Check sheet for the modelled part. Datum: model origin and axes. Units: mm. A direction names the side the tool comes from. Round coordinates to 2 decimals unless told otherwise and drop trailing zeros. Order: outer loops, then holes, each group sorted by start corner. A loop starts at its lowest first (then second) coordinate and runs counter-clockwise, first axis right, second up.
```python
from build123d import *

# Parameters (mm, degrees)
BOSS_EXTRUDE1_DEPTH = 3
SKETCH3_W           = 5
SKETCH3_H           = 3
CUT_EXTRUDE2_DEPTH  = 55.166410256
SKETCH4_W           = 3
SKETCH4_H           = 15
CUT_EXTRUDE3_DEPTH  = 55.166410256
SKETCH5_R           = 1.5
CUT_EXTRUDE4_DEPTH  = 55.166410256
SKETCH6_R           = 1.6
CUT_EXTRUDE5_DEPTH  = 55.166410256


with BuildPart() as part:
    # Sketch1 → Boss-Extrude1 (new body)
    with BuildSketch(Plane(origin=(0, 0, 0), x_dir=(1, 0, 0), z_dir=(0, 1, 0))):
        Polygon((-45, 27), (-22.5, 27), (-22.5, 30), (-7.5, 30), (-7.5, 27), (7.5, 27), (7.5, 30), (22.5, 30), (22.5, 27), (45, 27), (45, -27), (22.5, -27), (22.5, -30), (7.5, -30), (7.5, -27), (-7.5, -27), (-7.5, -30), (-22.5, -30), (-22.5, -27), (-45, -27), align=None)
    extrude(amount=BOSS_EXTRUDE1_DEPTH)

    # Sketch3 → Cut-Extrude2 (cut, through all)
    with BuildSketch(Plane(origin=(0, 3, 0), x_dir=(1, 0, 0), z_dir=(0, 1, 0))):
        with Locations((-34.25, -19.5)):
            Rectangle(SKETCH3_W, SKETCH3_H)
        with Locations((-36.79, 19.5)):
            Rectangle(SKETCH3_W, SKETCH3_H)
    extrude(amount=-CUT_EXTRUDE2_DEPTH, mode=Mode.SUBTRACT)

    # Sketch4 → Cut-Extrude3 (cut, through all)
    with BuildSketch(Plane(origin=(0, 3, 0), x_dir=(1, 0, 0), z_dir=(0, 1, 0))):
        Rectangle(SKETCH4_W, SKETCH4_H)
    extrude(amount=-CUT_EXTRUDE3_DEPTH, mode=Mode.SUBTRACT)

    # Sketch5 → Cut-Extrude4 (cut, through all)
    with BuildSketch(Plane(origin=(0, 3, 0), x_dir=(1, 0, 0), z_dir=(0, 1, 0))):
        with Locations(Location((39, 8, 0), (0, 0, 270))):
            Circle(SKETCH5_R)
    extrude(amount=-CUT_EXTRUDE4_DEPTH, mode=Mode.SUBTRACT)

    # Sketch6 → Cut-Extrude5 (cut, through all)
    with BuildSketch(Plane(origin=(0, 3, 0), x_dir=(1, 0, 0), z_dir=(0, 1, 0))):
        with Locations(Location((-28.1, 18.35, 0), (0, 0, 270))):
            Circle(SKETCH6_R)
        with Locations(Location((-28.1, 0.65, 0), (0, 0, 270))):
            Circle(SKETCH6_R)
    extrude(amount=-CUT_EXTRUDE5_DEPTH, mode=Mode.SUBTRACT)


solid = part.part
```
Item 1: Sectioned sample at C-C (x = -28.1). Record the cut outline in (y, z).
Answer:
outline: (0, -27) - (3, -27) - (3, -19.95) - (0, -19.95) - close; (0, -16.75) - (3, -16.75) - (3, -2.25) - (0, -2.25) - close; (0, 0.95) - (3, 0.95) - (3, 27) - (0, 27) - close
Item 2: Sectioned sample at B-B (x = 39). Record the cut outline in (y, z).
Answer:
outline: (0, -27) - (3, -27) - (3, -9.5) - (0, -9.5) - close; (0, -6.5) - (3, -6.5) - (3, 27) - (0, 27) - close
Item 3: Sectioned sample at D-D (y = 0.45). State how many separate pieces and enclosed holes the cut face has, and give its area (3 significant figures).
Answer:
separate pieces: 1
enclosed holes: 6
area: 4,940 mm2
Item 4: Go/stop test with flat-tipped pins: P1, Ø0.9, axis at y = 1.5, z = 28, coming from the +X side; P2, Ø1.5, axis at y = 1.5, z = -29, coming from the -X side; P3, Ø3.5, axis at x = 39, z = -8, coming from the +Y side; P4, Ø0.9, axis at x = -2.5, y = 1.5, coming from the -Z side. Record where each tip stops, or that it passes through.
Answer:
P1: stops at x = 22.5
P2: stops at x = -22.5
P3: stops at y = 3
P4: stops at z = -27
Item 5: Access from +Z, -Z, +X, -X, +Y, -Y to the whole of each face (thin tool, end or side, straight path). Record for faces 4 (the flat face through (-1.5, 2, 0)), 5 (the flat face through (22.5, 1, 28)), 6 (the flat face through (34, 1, -27)), 7 (the flat face through (-34, 1, 27)), 8 (the flat face through (-34, 1, -27)).
Answer:
face 4: +Y, -Y
face 5: +Z, +X, +Y, -Y
face 6: -Z, +X, +Y, -Y
face 7: +Z, -X, +Y, -Y
face 8: -Z, -X, +Y, -Y
Item 6: Scan lines: line 1 along X through (y, z) = (1.7, -18.35); line 2 along X through (y, z) = (2.8, 5); line 3 along X through (y, z) = (1.1, -8). Record each from-to range of solid material in increasing order.
Answer:
line 1: x = -45 to -39.29, -34.29 to -29.7, -26.5 to 45
line 2: x = -45 to -1.5, 1.5 to 45
line 3: x = -45 to 37.5, 40.5 to 45
Item 7: Release check for a two-part mould opening along Z. For faces 1 (the flat face through (-39.29, 2, -19)), 2 (the flat face through (11, 3, 0)), 3 (the flat face through (15, 1, 30)) record: released by +Z, released by -Z, zero draft, split by the parting line, or undercut.
Answer:
face 1: undercut
face 2: zero draft
face 3: released by +Z
Item 8: Sectioned sample at A-A (z = -4.5). Record the cut outline in (x, y).
Answer:
outline: (-45, 0) - (-1.5, 0) - (-1.5, 3) - (-45, 3) - close; (1.5, 0) - (45, 0) - (45, 3) - (1.5, 3) - close
